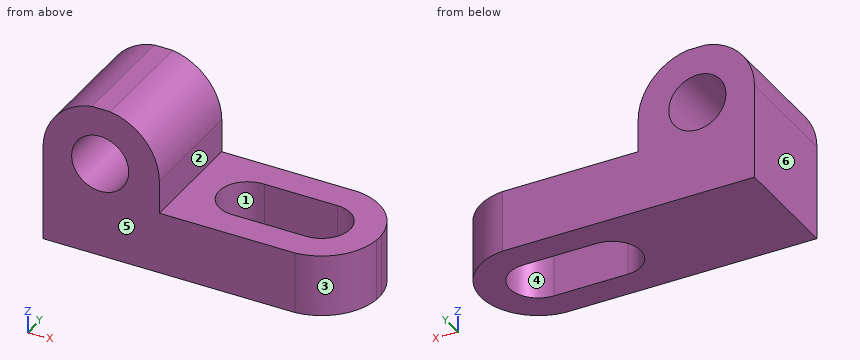
```python
from build123d import *

# Parameters (mm, degrees)
F1_DEPTH = 25.4
F3_DEPTH = 50.8
F4_R     = 6.35
F5_DEPTH = 13.7715663219
F7_DEPTH = 13.7715663219
F9_DEPTH = 13.7715663219


with BuildPart() as f1:
    # F0 (on Front) → F1 (new body)
    with BuildSketch(Plane.XZ):
        Polygon((0, 33.8735803962), (0, 0), (67.6466450095, 0), (67.6466450095, 13.7705663219), (25.8323773742, 13.7705663219), (25.8323773742, 33.8735803962), align=None)
    extrude(amount=F1_DEPTH)

    # F2 (on face) → F3 (cut)
    with BuildSketch(Plane.XZ.offset(25.4)):
        with BuildLine():
            Line((0, 33.8735803962), (0, 21.1735803962))
            ThreePointArc((0, 21.1735803962), (3.0977100292, 29.5149442417), (10.8550581005, 33.8735803962))
            Line((10.8550581005, 33.8735803962), (0, 33.8735803962))
        make_face()
        with BuildLine():
            ThreePointArc((19.05, 21.1735803962), (12.7, 27.5235803962), (6.35, 21.1735803962))
            Line((6.35, 21.1735803962), (12.7, 21.1735803962))
            Line((12.7, 21.1735803962), (19.05, 21.1735803962))
        make_face()
        with BuildLine():
            Line((12.7, 21.1735803962), (6.35, 21.1735803962))
            ThreePointArc((6.35, 21.1735803962), (12.7, 14.8235803962), (19.05, 21.1735803962))
            Line((19.05, 21.1735803962), (12.7, 21.1735803962))
        make_face()
        with BuildLine():
            Line((25.8323773742, 33.8735803962), (14.9773192737, 33.8735803962))
            ThreePointArc((14.9773192737, 33.8735803962), (22.734667345, 29.5149442417), (25.8323773742, 21.1735803962))
            Line((25.8323773742, 21.1735803962), (25.8323773742, 33.8735803962))
        make_face()
    extrude(amount=-F3_DEPTH, mode=Mode.SUBTRACT)

    # F4 (on face) → F5 (cut, through all)
    with BuildSketch(Plane.XY.offset(13.7705663219)):
        with Locations((38.5323773742, -12.7)):
            Circle(F4_R)
        with Locations((54.9466450095, -12.7)):
            Circle(F4_R)
    extrude(amount=-F5_DEPTH, mode=Mode.SUBTRACT)

    # F6 (on face) → F7 (cut, through all)
    with BuildSketch(Plane.XY.offset(13.7705663219)):
        with BuildLine():
            Line((54.9441526312, -6.3500004891), (38.8158588696, -6.3563308534))
            ThreePointArc((38.8158588696, -6.3563308534), (43.121636982, -8.3112420605), (44.8823773742, -12.7))
            ThreePointArc((44.8823773742, -12.7), (43.0225055016, -17.1901279936), (38.5323775634, -19.05))
            Line((38.5323775634, -19.05), (54.9441526312, -19.0499995109))
            ThreePointArc((54.9441526312, -19.0499995109), (48.5966450095, -12.7), (54.9441526312, -6.3500004891))
        make_face()
    extrude(amount=-F7_DEPTH, mode=Mode.SUBTRACT)

    # F8 (on face) → F9 (cut, through all)
    with BuildSketch(Plane.XY.offset(13.7705663219)):
        with BuildLine():
            ThreePointArc((55.9713775557, 0), (63.9560866346, -3.6905583749), (67.6466450095, -11.6752674539))
            Line((67.6466450095, -11.6752674539), (67.6466450095, 0))
            Line((67.6466450095, 0), (55.9713775557, 0))
        make_face()
        with BuildLine():
            Line((67.6466450095, -25.4), (67.6466450095, -13.7247325461))
            ThreePointArc((67.6466450095, -13.7247325461), (63.9560866346, -21.7094416251), (55.9713775557, -25.4))
            Line((55.9713775557, -25.4), (67.6466450095, -25.4))
        make_face()
        with BuildLine():
            Line((53.9219124634, 0), (55.9713775557, 0))
            ThreePointArc((55.9713775557, 0), (54.9466450095, 0.0412745356), (53.9219124634, 0))
        make_face()
    extrude(amount=-F9_DEPTH, mode=Mode.SUBTRACT)


solid = f1.part
```
CAD build for the part. Positions are in the model's coordinates, mm. Face numbers are marked on the shaded views. A direction names the side the tool comes from. Round coordinates to 2 decimals unless told otherwise and drop trailing zeros. Write each loop counter-clockwise with the first axis right and the second up, starting at its lowest first coordinate (ties: lowest second). Pieces come first, ordered by that corner, then holes. Notation, with made-up numbers: (68.5, -35.5) -> (101.5, -35.5) arc R21 cw to (101.5, -16.5) -> close; hole circle Ø11 at (-21, 10). An arc over 180 degrees is marked (long way). Answer in a Markdown table with one row per item. Add a question column.
Item 1: Mould opens along Y. For the marked faces 4, 5 and 6 say: pulls with the +Y half, pulls with the -Y half, needs draft (parallel to the pull), parting line crosses it, or undercut.
Item 2: Saw through at C-C, the plane z = 8.5. Write the cut outline in (x, y).
Item 3: Saw through at B-B, the plane x = 12.7. Write the cut outline in (y, z).
Item 4: Saw through at A-A, the plane y = -12.7. Write the cut outline in (x, z).
Item 5: Drill centre lines: line 1 (Z direction, x = 12.7, y = -5.25); line 2 (X direction, y = -10.5, z = 14); line 3 (Y direction, x = 34, z = 7). Where is each one in solid material? Low to high. Write a range as from..to.
Item 6: Drop flat-ended pins along their axis: pin 1 Ø10 at (x, y) = (53, -15) entering from +Z; pin 2 Ø10 at (x, z) = (30, 14.5) entering from -Y. Give the stop position or say it passes through.
Item 7: Saw through at D-D, the plane y = -17.5. Write the cut outline in (x, z), then the cut area to 3 significant figures.
Item 8: Which spindle directions (+Z, -Z, +X, -X, +Y, -Y) get a long thin tool onto all of the face, cutting with end or side? Do the marked faces 1, 2 and 3. Say none if no direction does.
Findings below:
| question | item | result |
|---|---|---|
| 1 | face 4 | undercut |
| 1 | face 5 | pulls with the -Y half |
| 1 | face 6 | needs draft |
| 2 | outline | (0, -25.4) -> (55.97, -25.4) arc R12.74 ccw to (67.65, -13.72) -> (67.65, -11.68) arc R12.74 ccw to (55.97, 0) -> (0, 0) -> close; hole (38.53, -19.05) -> (54.94, -19.05) arc R6.35 ccw to (54.94, -6.35) -> (38.82, -6.36) arc R6.35 ccw (long way) to start |
| 3 | outline | (-25.4, 0) -> (0, 0) -> (0, 14.82) -> (-25.4, 14.82) -> close; (-25.4, 27.52) -> (0, 27.52) -> (0, 33.87) -> (-25.4, 33.87) -> close |
| 4 | outline | (0, 0) -> (32.18, 0) -> (32.18, 13.77) -> (25.83, 13.77) -> (25.83, 21.17) arc R12.92 ccw to (14.98, 33.87) -> (10.86, 33.87) arc R12.92 ccw to (0, 21.17) -> close; (61.3, 0) -> (67.65, 0) -> (67.65, 13.77) -> (61.3, 13.77) -> close; hole circle Ø12.7 at (12.7, 21.17) |
| 5 | line 1 | z = 0..14.82, 27.52..33.87 |
| 5 | line 2 | x = 0..25.83 |
| 5 | line 3 | y = -25.4..-17.15, -8.25..0 |
| 6 | pin 1 | stops at z = 13.77 |
| 6 | pin 2 | stops at y = -25.4 |
| 7 | outline | (0, 0) -> (34.38, 0) -> (34.38, 13.77) -> (25.83, 13.77) -> (25.83, 21.17) arc R12.92 ccw to (14.98, 33.87) -> (10.86, 33.87) arc R12.92 ccw to (0, 21.17) -> close; (59.1, 0) -> (66.75, 0) -> (66.75, 13.77) -> (59.1, 13.77) -> close; hole circle Ø12.7 at (12.7, 21.17) |
| 7 | area | 903 mm^2 |
| 8 | face 1 | +Z, -Z |
| 8 | face 2 | +Z, +X, +Y, -Y |
| 8 | face 3 | +Z, -Z, +X, -Y |
